The drawing under review shows one solid part. Ordinate dimensions are in mm from its lowest x, y, z. Round coordinates to 2 decimals unless told otherwise and drop trailing zeros. Write each loop counter-clockwise with the first axis right and the second up, starting at its lowest first coordinate (ties: lowest second). Pieces come first, ordered by that corner, then holes. Notation, with made-up numbers: (28, 60) -> (57, 60) arc R16 cw to (57, 82) -> close; hole circle Ø9 at (83.25, -21.75). An arc over 180 degrees is marked (long way). Write item = value, one per line. Start each with the question number.
Item 1: Add section C-C, the plane z = 35. State the section outline as (x, y) points.
Item 2: For pin 1 Ø2 at (x, z) = (80.7, 93.05) entering from -Y; pin 2 Ø1.5 at (x, y) = (18, 2) entering from -Z; pin 3 Ø4 at (x, z) = (50, 94.3) entering from -Y; pin 4 Ø1.5 at (y, z) = (2, 89) entering from -X, all flat-tipped, find the tip position at first contact; note any pin that passes through.
Item 3: Add section D-D, the plane x = 50. State the section outline as (y, z) points, then the cut area to 3 significant figures.
Item 4: Add section A-A, the plane x = 80.7. State the section outline as (y, z) points.
Item 5: To check wall thickness, follow L1, parallel to X at y = 2, z = 74.95; L2, parallel to Z at x = 6, y = 2.3; L3, parallel to Z at x = 32, y = 1.75. State the ranges of each line that lie inside material, in increasing order.
Item 6: Add section B-B, the plane y = 1.6. State how many separate pieces and enclosed holes the cut face has, then the cut area to 3 significant figures.
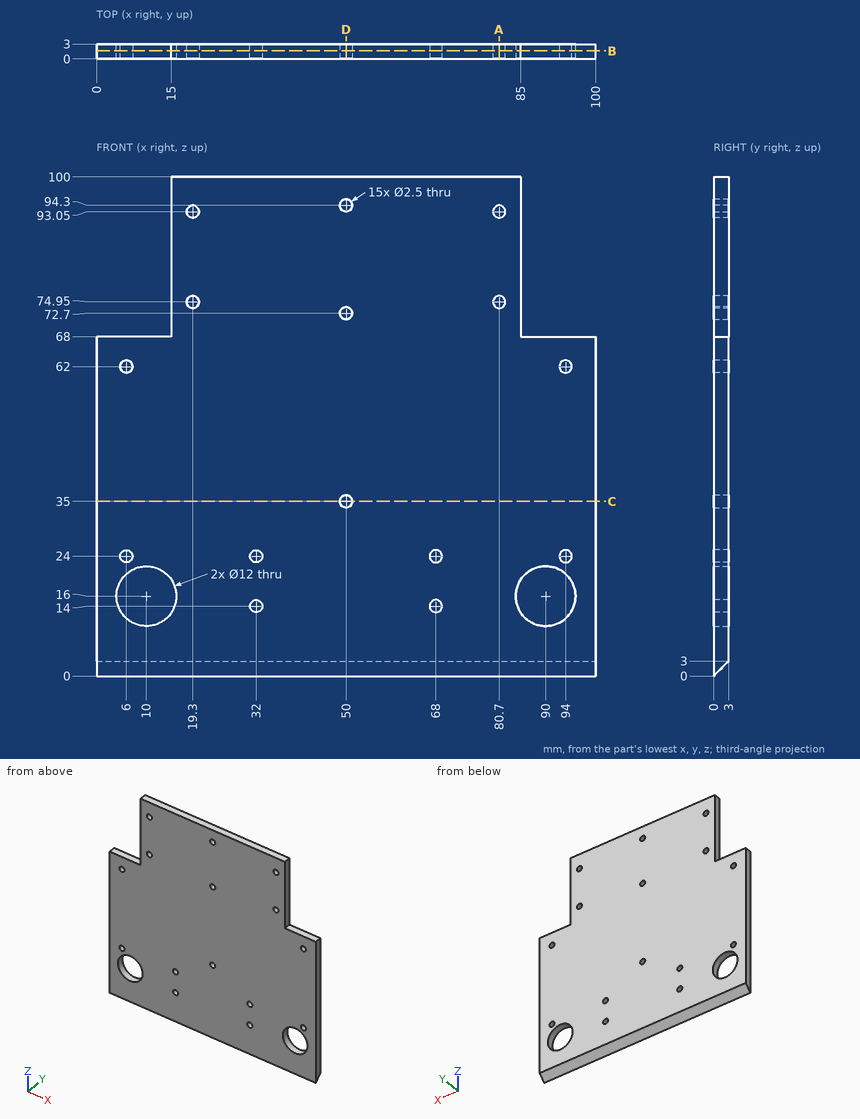
Result set:
q1.outline = (0, 0) -> (48.75, 0) -> (48.75, 3) -> (0, 3) -> close; (51.25, 0) -> (100, 0) -> (100, 3) -> (51.25, 3) -> close
q2.pin_1 = through
q2.pin_2 = 1.25
q2.pin_3 = 0
q2.pin_4 = 15
q3.outline = (0, 0) -> (3, 3) -> (3, 33.75) -> (0, 33.75) -> close; (0, 36.25) -> (3, 36.25) -> (3, 71.45) -> (0, 71.45) -> close; (0, 73.95) -> (3, 73.95) -> (3, 93.05) -> (0, 93.05) -> close; (0, 95.55) -> (3, 95.55) -> (3, 100) -> (0, 100) -> close
q3.area = 273 mm²
q4.outline = (0, 0) -> (3, 3) -> (3, 73.7) -> (0, 73.7) -> close; (0, 76.2) -> (3, 76.2) -> (3, 91.8) -> (0, 91.8) -> close; (0, 94.3) -> (3, 94.3) -> (3, 100) -> (0, 100) -> close
q5.L1 = 15 to 18.05, 20.55 to 79.45, 81.95 to 85
q5.L2 = 2.3 to 11.53, 20.47 to 22.75, 25.25 to 60.75, 63.25 to 68
q5.L3 = 1.75 to 12.75, 15.25 to 22.75, 25.25 to 100
q6.separate_pieces = 1
q6.enclosed_holes = 17
q6.area = 8,580 mm²
